Read the model definition and answer for the solid it produces. Units are mm, in the model's axes. Face numbers are marked on the shaded views. Coordinates: 2 decimals unless noted, no trailing zeros. Write each loop counter-clockwise with the first axis right and the second up, starting at its lowest first coordinate (ties: lowest second). Pieces come first, ordered by that corner, then holes.
from build123d import *

# Parameters (mm, degrees)
SKETCH1_R                = 0.95
BOSS_EXTRUDE1_DEPTH      = 18
FILLET1_R                = 2
CUT_EXTRUDE1_DEPTH       = 83.510909783
CUT_EXTRUDE1_DEPTH_BACK  = 83.510909783
SKETCH2_W                = 32
SKETCH2_H                = 82.41
BOSS_EXTRUDE2_DEPTH      = 18
BOSS_EXTRUDE2_DEPTH_BACK = 16
SKETCH3_R                = 3.75


with BuildPart() as part:
    # Sketch1 → Boss-Extrude1 (new, symmetric)
    with BuildSketch(Plane(origin=(0, 0, 0), x_dir=(0, 0, -1), z_dir=(1, 0, 0))):
        with BuildLine():
            Line((0, 3.13), (31.1, 3.13))
            Line((31.1, 3.13), (46.5, 1.782674582))
            Line((46.5, 1.782674582), (63, -0.639122384))
            Line((63, -0.639122384), (70.830854785, -5.891324783))
            ThreePointArc((70.830854785, -5.891324783), (73.097482442, -6.811154728), (75.542872081, -6.749855612))
            Line((75.542872081, -6.749855612), (76.479440337, -6.530221264))
            ThreePointArc((76.479440337, -6.530221264), (79.183707452, -8.094392066), (77.788191978, -10.889428289))
            Line((77.788191978, -10.889428289), (70.085210842, -13.7273023))
            ThreePointArc((70.085210842, -13.7273023), (67.51150317, -14.076398492), (65.031397439, -13.305091226))
            Line((65.031397439, -13.305091226), (61.593330792, -11.338037731))
            ThreePointArc((61.593330792, -11.338037731), (60.042423522, -10.718485849), (58.380824128, -10.550422334))
            Line((58.380824128, -10.550422334), (37.261773194, -11.370750671))
            ThreePointArc((37.261773194, -11.370750671), (36.078702039, -10.834444885), (35.799894202, -9.565765476))
            Line((35.799894202, -9.565765476), (36.542469609, -6.634487021))
            ThreePointArc((36.542469609, -6.634487021), (36.281163577, -5.387851181), (35.136870597, -4.828409195))
            Line((35.136870597, -4.828409195), (7, -4.828409195))
            Line((7, -4.828409195), (-0.7040968, -3.049778303))
            ThreePointArc((-0.7040968, -3.049778303), (-3.109879908, 0.354326059), (0, 3.13))
        make_face()
        Circle(SKETCH1_R, mode=Mode.SUBTRACT)
        with Locations((44.1, -5.6)):
            Circle(SKETCH1_R, mode=Mode.SUBTRACT)
        with Locations((39.75, -8.75)):
            Circle(SKETCH1_R, mode=Mode.SUBTRACT)
        with Locations((77, -8.75)):
            Circle(SKETCH1_R, mode=Mode.SUBTRACT)
    extrude(amount=BOSS_EXTRUDE1_DEPTH, both=True)

    # Fillet1
    # the kernel refuses this fillet: 2 mm, written as the material it takes off along each edge
    with BuildSketch(Plane(origin=(19.131384491, -0.639122384, -63), x_dir=(0, -0.557020574337694, -0.8304986934152909), z_dir=(-1, 0, 0))) as fillet1_piece_1:
        with BuildLine():
            CenterArc((FILLET1_R * 0.226276898255, FILLET1_R), FILLET1_R, 244.5, 25.5)
            Line((-FILLET1_R * 0.204234198553, FILLET1_R * 0.0974147156501), (0, 0))
            Line((0, 0), (FILLET1_R * 0.226276898255, 0))
        make_face()
    extrude(amount=38.262768983, mode=Mode.SUBTRACT)
    with BuildSketch(Plane(origin=(-18.569678042, -4.828409195, -7), x_dir=(0, 0.22495105434386356, 0.9743700647852356), z_dir=(1, 0, 0))) as fillet1_piece_2:
        with BuildLine():
            CenterArc((FILLET1_R * 0.113935608302, -FILLET1_R), FILLET1_R, 90, 13)
            Line((-FILLET1_R * 0.111015446042, -FILLET1_R * 0.0256299352148), (0, 0))
            Line((0, 0), (FILLET1_R * 0.113935608302, 0))
        make_face()
    extrude(amount=37.139356083, mode=Mode.SUBTRACT)
    with BuildSketch(Plane(origin=(18.218304715, 3.13, -31.1), x_dir=(0, 0, 1), z_dir=(-1, 0, 0))) as fillet1_piece_3:
        with BuildLine():
            CenterArc((FILLET1_R * 0.0436609429085, -FILLET1_R), FILLET1_R, 90, 5)
            Line((-FILLET1_R * 0.0434947998391, -FILLET1_R * 0.00380530190825), (0, 0))
            Line((0, 0), (FILLET1_R * 0.0436609429085, 0))
        make_face()
    extrude(amount=36.436609429, mode=Mode.SUBTRACT)
    with BuildSketch(Plane(origin=(18.14621298, 1.782674582, -46.5), x_dir=(0, -0.14521967007723557, -0.9893994377513355), z_dir=(-1, 0, 0))) as fillet1_piece_4:
        with BuildLine():
            CenterArc((FILLET1_R * 0.0292425960983, FILLET1_R), FILLET1_R, 266.65, 3.35)
            Line((-FILLET1_R * 0.02919262642, FILLET1_R * 0.00170879761001), (0, 0))
            Line((0, 0), (FILLET1_R * 0.0292425960983, 0))
        make_face()
    extrude(amount=36.292425961, mode=Mode.SUBTRACT)

    # Sketch2 → Cut-Extrude1 (cut, two sides: drawn at the far end of the back side and taken through both)
    with BuildSketch(Plane(origin=(0, 0, 0), x_dir=(1, 0, 0), z_dir=(0, 1, 0)).offset(-CUT_EXTRUDE1_DEPTH_BACK)):
        with Locations((0, 38.075)):
            Rectangle(SKETCH2_W, SKETCH2_H)
    extrude(amount=CUT_EXTRUDE1_DEPTH + CUT_EXTRUDE1_DEPTH_BACK, mode=Mode.SUBTRACT)


with BuildPart() as cut_extrude1_piece_1:
    # of the separate pieces the step leaves, piece 1, a body of its own (cut_extrude1_pieces)
    add(part.part.solids().sort_by_distance((16, 3.13, 0))[0])



with BuildPart() as cut_extrude1_piece_2:
    # of the separate pieces the step leaves, piece 2, a body of its own (cut_extrude1_pieces)
    add(part.part.solids().sort_by_distance((-18, 3.13, 0))[0])


with BuildPart() as cut_extrude1_piece_1_1:
    add(cut_extrude1_piece_1.part)

    add(cut_extrude1_piece_2.part)  # Boss-Extrude2 merges Cut-Extrude1 piece 2
    # Sketch3 → Boss-Extrude2 (add, two sides: drawn at the far end of the back side and taken through both)
    with BuildSketch(Plane(origin=(0, 0, 0), x_dir=(0, 0, -1), z_dir=(1, 0, 0)).offset(-BOSS_EXTRUDE2_DEPTH_BACK)):
        with Locations((58.65, -5.75)):
            Circle(SKETCH3_R)
    extrude(amount=BOSS_EXTRUDE2_DEPTH + BOSS_EXTRUDE2_DEPTH_BACK)


solid = cut_extrude1_piece_1_1.part
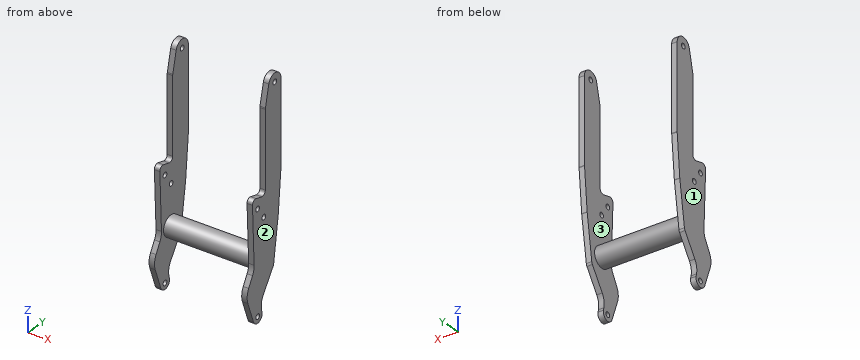
Item 1: The part is cut by section A-A (z = -10). Give the vertices of the cut face in (x, y).
Item 2: The part is cut by section C-C (x = -14). Give the vertices of the cut face in (y, z).
Item 3: The part is cut by section B-B (z = -44.1). Give the vertices of the cut face in (x, y).
Item 4: Find the intervals of material crossed by probe 1 along X at (y, z) = (-1.25, -46.5); probe 2 along Z at (x, y) = (17.15, -8.75); probe 3 along Y at (x, z) = (16.9, -39.75), in increasing order.
Item 5: Determine the mould class of the marked faces 1, 2 and 3 for opening direction X: +X half, -X half, draft (parallel to the pull), parting line (faces both ways), or undercut.
Item 6: Given pin 1 (10 mm diameter, centred on x = 11.5, y = -11, fed in from -Z); pin 2 (1 mm diameter, centred on x = -17.5, z = -14.5, fed in from -Y); pin 3 (3 mm diameter, centred on y = 1, z = -66, fed in from -X); pin 4 (12 mm diameter, centred on x = 0.5, z = -49.5, fed in from -Y), each flat-ended and moving along its own axis, determine where each tip first touches the part or whether it passes through.
Item 7: The part is cut by section D-D (z = -73.5). Give the vertices of the cut face in (x, y).
Answer:
1. outline: (-18, -4.83) - (-16, -4.83) - (-16, 3.13) - (-18, 3.13) - close; (16, -4.83) - (18, -4.83) - (18, 3.13) - (16, 3.13) - close
2. outline: circle Ø7.5 at (-5.75, -58.65)
3. outline: (-18, -11.11) - (-16, -11.11) - (-16, -6.55) - (-18, -6.55) - close; (-18, -4.65) - (-16, -4.65) - (-16, 1.99) - (-18, 1.99) - close; (16, -11.11) - (18, -11.11) - (18, -6.55) - (16, -6.55) - close; (16, -4.65) - (18, -4.65) - (18, 1.99) - (16, 1.99) - close
4. probe 1: x = -18 to -16, 16 to 18
4. probe 2: z = -79.28 to -77.95, -76.05 to -40.7, -38.8 to -36.01
4. probe 3: y = -11.27 to -9.7, -7.8 to 2.37
5. face 1: -X half
5. face 2: +X half
5. face 3: undercut
6. pin 1: stops at z = -79.28
6. pin 2: stops at y = -4.83
6. pin 3: passes through
6. pin 4: stops at y = -7.78
7. outline: (-18, -12.47) - (-16, -12.47) - (-16, -6.87) - (-18, -6.87) - close; (16, -12.47) - (18, -12.47) - (18, -6.87) - (16, -6.87) - close
